from build123d import *

# Parameters (mm, degrees)
SKETCH1_W                          = 107.95
SKETCH1_H                          = 12.7
BOSS_EXTRUDE1_DEPTH                = 29.36875
TAP_DRILL_FOR_8_32_TAP1_AT_2_COUNT = 2
TAP_DRILL_FOR_8_32_TAP1_AT_2_PITCH = 76.2
TAP_DRILL_FOR_8_32_TAP1_AT_3_COUNT = 2
TAP_DRILL_FOR_8_32_TAP1_AT_3_PITCH = 38.1
FILLET1_R                          = 1.5875


with BuildPart() as part:
    # Sketch1 → Boss-Extrude1 (new, symmetric)
    with BuildSketch(Plane.XY):
        Rectangle(SKETCH1_W, SKETCH1_H)
    extrude(amount=BOSS_EXTRUDE1_DEPTH, both=True)

    # Sketch4 → Tap Drill for #8-32 Tap1 (revolve, cut)
    with BuildSketch(Plane(origin=(-38.1, 0, 29.36875), x_dir=(0, -1, 0), z_dir=(1, 0, 0))):
        Polygon((0, 0), (0, 20.087806461), (1.7272, 19.05), (1.7272, 0), align=None)
    tap_drill_for_8_32_tap1 = revolve(axis=Axis((-38.1, 0, 35.71875), (0, 0, -1)), mode=Mode.SUBTRACT)

    # Tap Drill for #8-32 Tap1 at 2: Tap Drill for #8-32 Tap1 ×2
    with Locations(*[(i * TAP_DRILL_FOR_8_32_TAP1_AT_2_PITCH, 0, 0) for i in range(1, TAP_DRILL_FOR_8_32_TAP1_AT_2_COUNT)]):
        add(tap_drill_for_8_32_tap1, mode=Mode.SUBTRACT)

    # Tap Drill for #8-32 Tap1 at 3: Tap Drill for #8-32 Tap1 ×2
    with Locations(*[(i * TAP_DRILL_FOR_8_32_TAP1_AT_3_PITCH, 0, 0) for i in range(1, TAP_DRILL_FOR_8_32_TAP1_AT_3_COUNT)]):
        add(tap_drill_for_8_32_tap1, mode=Mode.SUBTRACT)

    # Mirror1: Tap Drill for #8-32 Tap1 across plane
    add(tap_drill_for_8_32_tap1.mirror(Plane.XY), mode=Mode.SUBTRACT)

    # Mirror1 copy 1 sketch → Mirror1 copy 1 (revolve, cut)
    with BuildSketch(Plane(origin=(38.1, 0, -29.36875), x_dir=(0, -1, 0), z_dir=(1, 0, 0))):
        Polygon((0, 0), (0, -20.087806461), (1.7272, -19.05), (1.7272, 0), align=None)
    revolve(axis=Axis((38.1, 0, -35.71875), (0, 0, -1)), mode=Mode.SUBTRACT)

    # Mirror1 copy 2 sketch → Mirror1 copy 2 (revolve, cut)
    with BuildSketch(Plane(origin=(0, 0, -29.36875), x_dir=(0, -1, 0), z_dir=(1, 0, 0))):
        Polygon((0, 0), (0, -20.087806461), (1.7272, -19.05), (1.7272, 0), align=None)
    revolve(axis=Axis((0, 0, -35.71875), (0, 0, -1)), mode=Mode.SUBTRACT)

    # Fillet1
    fillet1_edges = [part.edges().sort_by_distance(p)[0] for p in [
        (-53.975, 6.35, 0),
        (53.975, 6.35, 0),
    ]]
    fillet(fillet1_edges, radius=FILLET1_R)


solid = part.part
Check sheet for the modelled part. Datum: model origin and axes. Units: mm. A direction names the side the tool comes from. Give positions to 0.01 mm unless a question says otherwise; leave off trailing zeros. One line per item, written item: value. Start each with the question number.
Item 1: Section check A-A on z = 24.5. State how many separate pieces and enclosed holes the cut face has, then the cut area to 3 significant figures.
Item 2: Tool access check on faces 4 (the flat face through (-1, -6.35, 0)), 5 (the cylindrical face through (1.05, 1.37, 19.98)), 6 (the cylindrical face through (36.387, 0.225, -19.977)). Record the directions out of +Z, -Z, +X, -X, +Y, -Y that give a thin tool (end or side, any length) a straight path to the whole face; none if there is none.
Item 3: Material ranges on probe 1 along X at (y, z) = (0, 15.25) (3 decimals); probe 2 along Y at (x, z) = (-38, 20); probe 3 along X at (y, z) = (-0.75, 25.5) (3 decimals), recorded low to high. Write a range as from..to.
Item 4: Gauge pin test, flat ends, axial feed: pin 1 (5.5 mm diameter, centred on x = 38.1, y = 0, fed in from +Z); pin 2 (3 mm diameter, centred on x = 0, y = 0, fed in from +Z); pin 3 (2 mm diameter, centred on x = -38.1, y = 0, fed in from +Z); pin 4 (2 mm diameter, centred on x = 38.1, y = 0, fed in from -Z). Record the tip position at first contact, or that the pin passes through.
Item 5: Draft check along Y on faces 1 (the flat face through (-53.975, -1, 0)), 2 (the cylindrical face through (-36.414, 0.374, 19.977)), 3 (the flat face through (-1, 6.35, 0)). Enter one of: +Y half, -Y half, draft (parallel to the pull), parting line (faces both ways), or undercut.
Results list:
1. separate pieces: 1
1. enclosed holes: 3
1. area: 1,340 mm²
2. face 4: +Z, -Z, +X, -X, -Y
2. face 5: +Z
2. face 6: -Z
3. probe 1: -53.975..-39.827, -36.373..-1.727, 1.727..36.373, 39.827..53.975
3. probe 2: -6.35..-1.72, 1.72..6.35
3. probe 3: -53.975..-39.656, -36.544..-1.556, 1.556..36.544, 39.656..53.975
4. pin 1: z = 29.37
4. pin 2: z = 10.18
4. pin 3: z = 9.88
4. pin 4: z = -9.88
5. face 1: draft
5. face 2: undercut
5. face 3: +Y half
